```python
from build123d import *

# Parameters (mm, degrees)
SKETCH1_W           = 350
SKETCH1_H           = 300
SKETCH1_R           = 2
SKETCH1_R_2         = 3
SKETCH1_R_3         = 19
SKETCH1_R_4         = 2.5
BOSS_EXTRUDE1_DEPTH = 5
CUT_EXTRUDE1_REACH  = 232.543
SKETCH2_R           = 11
SKETCH2_R_2         = 9
SKETCH2_R_3         = 10
FILLET1_R           = 40
FILLET2_R           = 5
SKETCH3_R           = 12.5
SKETCH3_R_2         = 10
BOSS_EXTRUDE2_DEPTH = 15
SKETCH4_R           = 12.5
BOSS_EXTRUDE3_DEPTH = 2


with BuildPart() as part:
    # Sketch1 → Boss-Extrude1 (new body)
    with BuildSketch(Plane.XY):
        Rectangle(SKETCH1_W, SKETCH1_H)
        with Locations((-43.5, 75.344210129)):
            Circle(SKETCH1_R, mode=Mode.SUBTRACT)
        with Locations((43.5, 75.344210129)):
            Circle(SKETCH1_R, mode=Mode.SUBTRACT)
        with Locations((87, 0)):
            Circle(SKETCH1_R, mode=Mode.SUBTRACT)
        with Locations((43.5, -75.344210129)):
            Circle(SKETCH1_R, mode=Mode.SUBTRACT)
        with Locations((-43.5, -75.344210129)):
            Circle(SKETCH1_R, mode=Mode.SUBTRACT)
        with Locations((-87, 0)):
            Circle(SKETCH1_R, mode=Mode.SUBTRACT)
        with Locations((-76.012957941, -76.015)):
            Circle(SKETCH1_R_2, mode=Mode.SUBTRACT)
        with Locations((76.012957941, 76.015)):
            Circle(SKETCH1_R_2, mode=Mode.SUBTRACT)
        with Locations((76.012957941, -76.015)):
            Circle(SKETCH1_R_2, mode=Mode.SUBTRACT)
        with Locations((-76.012957941, 76.015)):
            Circle(SKETCH1_R_2, mode=Mode.SUBTRACT)
        with Locations((135, 0)):
            Circle(SKETCH1_R_3, mode=Mode.SUBTRACT)
        with Locations((158.55, -23.55)):
            Circle(SKETCH1_R_4, mode=Mode.SUBTRACT)
        with Locations((111.45, -23.55)):
            Circle(SKETCH1_R_4, mode=Mode.SUBTRACT)
        with Locations((111.45, 23.55)):
            Circle(SKETCH1_R_4, mode=Mode.SUBTRACT)
        with Locations((158.55, 23.55)):
            Circle(SKETCH1_R_4, mode=Mode.SUBTRACT)
    extrude(amount=BOSS_EXTRUDE1_DEPTH)

    # Sketch2 → Cut-Extrude1 (cut, up to next)
    with BuildSketch(Plane(origin=(0, 0, 0), x_dir=(-1, 0, 0), z_dir=(0, 0, -1)), mode=Mode.PRIVATE) as cut_extrude1_sk1:
        with Locations((-48.87, 15)):
            Circle(SKETCH2_R)
    cut_extrude1_tool1 = extrude(cut_extrude1_sk1.sketch, amount=-CUT_EXTRUDE1_REACH, mode=Mode.PRIVATE) & part.part
    # Sketch2 → Cut-Extrude1 (cut, up to next)
    with BuildSketch(Plane(origin=(0, 0, 0), x_dir=(-1, 0, 0), z_dir=(0, 0, -1)), mode=Mode.PRIVATE) as cut_extrude1_sk2:
        with Locations((-25, -50)):
            Circle(SKETCH2_R_2)
    cut_extrude1_tool2 = extrude(cut_extrude1_sk2.sketch, amount=-CUT_EXTRUDE1_REACH, mode=Mode.PRIVATE) & part.part
    # Sketch2 → Cut-Extrude1 (cut, up to next)
    with BuildSketch(Plane(origin=(0, 0, 0), x_dir=(-1, 0, 0), z_dir=(0, 0, -1)), mode=Mode.PRIVATE) as cut_extrude1_sk3:
        with Locations((-5, 50)):
            Circle(SKETCH2_R_3)
    cut_extrude1_tool3 = extrude(cut_extrude1_sk3.sketch, amount=-CUT_EXTRUDE1_REACH, mode=Mode.PRIVATE) & part.part
    add(cut_extrude1_tool1.solids().sort_by_distance((48.87, 15, 0))[0], mode=Mode.SUBTRACT)
    add(cut_extrude1_tool2.solids().sort_by_distance((25, -50, 0))[0], mode=Mode.SUBTRACT)
    add(cut_extrude1_tool3.solids().sort_by_distance((5, 50, 0))[0], mode=Mode.SUBTRACT)

    # Fillet1
    fillet1_edges = [part.edges().sort_by_distance(p)[0] for p in [
        (175, -150, 2.5),
        (-175, -150, 2.5),
        (-175, 150, 2.5),
        (175, 150, 2.5),
    ]]
    fillet(fillet1_edges, radius=FILLET1_R)

    # Fillet2
    fillet2_edges = [part.edges().sort_by_distance(p)[0] for p in [
        (163.284271247, 138.284271247, 0),
        (175, 0, 0),
        (163.284271247, -138.284271247, 0),
        (0, -150, 0),
        (-163.284271247, -138.284271247, 0),
        (-175, 0, 0),
        (-163.284271247, 138.284271247, 0),
        (0, 150, 0),
    ]]
    fillet(fillet2_edges, radius=FILLET2_R - 0.0001)  # a hair under: the kernel refuses the full size

    # Sketch3 → Boss-Extrude2 (add)
    with BuildSketch(Plane.XY.offset(5)):
        with Locations((5, 50)):
            Circle(SKETCH3_R)
        with Locations(Location((5, 50, 0), (0, 0, 180))):
            Circle(SKETCH3_R_2, mode=Mode.SUBTRACT)
    extrude(amount=BOSS_EXTRUDE2_DEPTH)

    # Sketch4 → Boss-Extrude3 (add)
    with BuildSketch(Plane.XY.offset(20)):
        with Locations((5, 50)):
            Circle(SKETCH4_R)
    extrude(amount=BOSS_EXTRUDE3_DEPTH)


solid = part.part
```
Work out the finished part from the listing and answer in its coordinate system (mm). A direction names the side the tool comes from. Give positions to 0.01 mm unless a question says otherwise; leave off trailing zeros.
(1) Which of the six approach directions +Z, -Z, +X, -X, +Y, -Y give full straight-line access (tool end or side, diameter ignored) to faces 4 (the cylindrical face through (20.16, -42.41, 2.46)), 5 (the flat face through (5, 50, 20))?
Final values:
face 4: +Z, -Z
face 5: -Z
(2) The part is cut by section C-C on y = 15. Count the separate pieces of the cut face and the enclosed holes in it, plus the area to 3 significant figures.
Final values:
separate pieces: 3
enclosed holes: 0
area: 1,510 mm2
(3) Straight lines are drawn through the part: line 1 (Y direction, x = 111.45, z = 3); line 2 (Z direction, x = 20, y = -12.5); line 3 (X direction, y = -12, z = 2.25). For each, find the intervals that lie inside material, in ascending order.
Final values:
line 1: y = -149.58 to -26.05, -21.05 to 21.05, 26.05 to 149.58
line 2: z = 0 to 5
line 3: x = -174.18 to 120.27, 149.73 to 174.18
(4) Flat-ended cylindrical pins translate along their axes: pin 1 Ø8 at (x, y) = (76.01, -76.02) entering from -Z; pin 2 Ø9.5 at (x, y) = (-76.01, 76.02) entering from +Z; pin 3 Ø1 at (x, z) = (-57.5, 6.5) entering from +Y; pin 4 Ø3 at (y, z) = (53, 15.5) entering from +X. Find the tip coordinate at first contact, or state that the pin passes through.
Final values:
pin 1: stops at z = 0
pin 2: stops at z = 5
pin 3: passes through
pin 4: stops at x = 17.41
(5) The mould has two halves that part along Y. Classify faces 1 (the flat face through (5, 50, 22)), 2 (the cylindrical face through (7.17, 59.76, 9.86)), 3 (the cylindrical face through (2.29, 37.797, 13.381)): pulls with the +Y half, pulls with the -Y half, needs draft (parallel to the pull), parting line crosses it, or undercut.
Final values:
face 1: needs draft
face 2: undercut
face 3: parting line crosses it
